from build123d import *

# Parameters (mm, degrees)
F0_W     = 76.2288123369
F0_H     = 76.380059123
F1_DEPTH = 76.2
F2_W     = 47.4917609245
F2_H     = 38.1900295615
F3_DEPTH = 76.2
F5_DEPTH = 76.2


with BuildPart() as f1:
    # F0 (on Front) → F1 (new body)
    with BuildSketch(Plane.XZ):
        with Locations((-38.1144061685, 38.1900295615)):
            Rectangle(F0_W, F0_H)
    extrude(amount=F1_DEPTH)

    # F2 (on face) → F3 (cut)
    with BuildSketch(Plane.XZ.offset(76.2)):
        with Locations((-52.4829318747, 57.2850443423)):
            Rectangle(F2_W, F2_H)
    extrude(amount=-F3_DEPTH, mode=Mode.SUBTRACT)

    # F4 (on face) → F5 (cut)
    with BuildSketch(Plane.XZ.offset(76.2)):
        Polygon((-76.2288123369, 0), (-28.7370514125, 38.1900295615), (-76.2288123369, 38.1900295615), align=None)
    extrude(amount=-F5_DEPTH, mode=Mode.SUBTRACT)


solid = f1.part
Here's how the part is built. I have some questions about the finished solid (model axes, mm). A direction names the side the tool comes from. Give positions to 0.01 mm unless a question says otherwise; leave off trailing zeros. Order: outer loops, then holes, each group sorted by start corner. A loop starts at its lowest first (then second) coordinate and runs counter-clockwise, first axis right, second up. Notation, with made-up numbers: (-6, -7) -> (43, -7) arc R23 ccw to (43, 10) -> close; hole circle Ø1 at (-24.5, -17.75). An arc over 180 degrees is marked (long way). Use a Markdown table: item, result. Add a question column.
Item 1: Imagine slicing it at C-C on x = -58.5. Please give me the cut outline in (y, z).
Item 2: Imagine slicing it at B-B on z = 71. Please give me the cut outline in (x, y).
Item 3: Imagine slicing it at A-A on y = -65. Please give me the cut outline in (x, z), plus the area to 3 significant figures.
Item 4: For faces 1 (the face through (-28.737, -39, 57)), 2 (the face through (-39, -38, 0)), which set-ups out of +Z, -Z, +X, -X, +Y, -Y let a thin tool reach every point of the face, with its end or its side?
Item 5: Will these pins go through, and if not, where does the flat tip stop? pin 1 (2 mm diameter, centred on y = -26.5, z = 51.5, fed in from -X); pin 2 (10 mm diameter, centred on x = -47, y = -35, fed in from +Z); pin 3 (8 mm diameter, centred on y = -39, z = 32.5, fed in from -X); pin 4 (4 mm diameter, centred on x = -16.5, z = 10.5, fed in from +Y).
Item 6: I need wall thicknesses on line 1 (X direction, y = -30, z = 70); line 2 (X direction, y = -21.5, z = 25); line 3 (Z direction, x = -36.5, y = -17). Which ranges of each line are inside material? Lowest first, please.
Data:
| question | item | result |
|---|---|---|
| 1 | outline | (-76.2, 0) -> (0, 0) -> (0, 14.26) -> (-76.2, 14.26) -> close |
| 2 | outline | (-28.74, -76.2) -> (0, -76.2) -> (0, 0) -> (-28.74, 0) -> close |
| 3 | outline | (-76.23, 0) -> (0, 0) -> (0, 76.38) -> (-28.74, 76.38) -> (-28.74, 38.19) -> close |
| 3 | area | 3,100 mm² |
| 4 | face 1 | +Z, -X, +Y, -Y |
| 4 | face 2 | -Z, +X, -X, +Y, -Y |
| 5 | pin 1 | stops at x = -28.74 |
| 5 | pin 2 | stops at z = 27.52 |
| 5 | pin 3 | stops at x = -40.79 |
| 5 | pin 4 | stops at y = 0 |
| 6 | line 1 | x = -28.74 to 0 |
| 6 | line 2 | x = -45.14 to 0 |
| 6 | line 3 | z = 0 to 31.95 |
